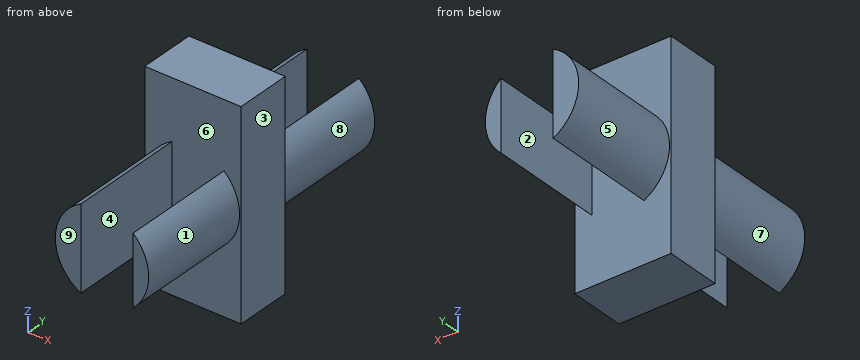
```python
from build123d import *

# Parameters (mm, degrees)
F1_DEPTH = 76.2
F2_W     = 29.7769960016
F2_H     = 106.9766134024
F3_DEPTH = 25.4


with BuildPart() as f1:
    # F0 (on Front) → F1 (new body, symmetric)
    with BuildSketch(Plane.XZ):
        with BuildLine():
            Line((-11.1479088664, -21.9459166651), (-11.1479088664, 21.9459166651))
            ThreePointArc((-11.1479088664, 21.9459166651), (-24.6150183905, 0), (-11.1479088664, -21.9459166651))
        make_face()
    extrude(amount=F1_DEPTH, both=True)



with BuildPart() as f1b:
    # F0 (on Front) → F1, piece 2 (new body, symmetric)
    with BuildSketch(Plane.XZ):
        with BuildLine():
            ThreePointArc((16.3939911872, -18.3612685651), (22.4659467298, -10.0588452567), (24.6150183905, 0))
            ThreePointArc((24.6150183905, 0), (22.4659467298, 10.0588452567), (16.3939911872, 18.3612685651))
            Line((16.3939911872, 18.3612685651), (16.3939911872, -18.3612685651))
        make_face()
    extrude(amount=F1_DEPTH, both=True)


with BuildPart() as f1_1:
    add(f1.part)

    add(f1b.part)  # F3 merges F1b
    # F2 (on Right) → F3 (join, symmetric)
    with BuildSketch(Plane.YZ):
        Rectangle(F2_W, F2_H)
    extrude(amount=F3_DEPTH, both=True)


solid = f1_1.part
```
The listing builds one solid part. Answer for the finished solid, in the listing's coordinates (mm). Face numbers are marked on the shaded views. A direction names the side the tool comes from. Coordinates: 2 decimals unless noted, no trailing zeros. Write each loop counter-clockwise with the first axis right and the second up, starting at its lowest first coordinate (ties: lowest second). Pieces come first, ordered by that corner, then holes. Notation, with made-up numbers: (-35, -6.5) - (-1, -6.5) arc R31 cw to (-1, 27.5) - close; hole circle Ø8 at (82.5, 81.5). An arc over 180 degrees is marked (long way). Return JSON: item names as keys, results as strings. Group by question number.
Q1. Flat-ended cylindrical pins translate along their axes: pin 1 Ø10 at (x, z) = (7, 5) entering from -Y; pin 2 Ø12 at (y, z) = (-48.5, 11) entering from -X; pin 3 Ø11 at (y, z) = (-42.5, -3) entering from -X (3 decimals). Find the tip coordinate at first contact, or state that the pin passes through.
Q2. Which of the six approach directions +Z, -Z, +X, -X, +Y, -Y give full straight-line access (tool end or side, diameter ignored) to the marked faces 1, 2, 3, 4 and 5?
Q3. For a pull along X with two mould halves and no side action, classify the marked faces 6, 7, 8 and 9 as +X half, -X half, draft (parallel to the pull), parting line (faces both ways), or undercut.
Q4. The part is cut by section D-D on z = 5.5. Write down the section's boundary in (x, y).
Q5. The part is cut by section B-B on x = 20. Write down the section's boundary in (y, z), and give its area (3 significant figures).
Q6. The part is cut by section A-A on z = -10.5. Write down the section's boundary in (x, y), and give its area (3 significant figures).
Q7. Find the intervals of material crossed by line 1 along Y through (x, z) = (5, -31.5); line 2 along X through (y, z) = (15, 6); line 3 along X through (y, z) = (-33, -21.5), in increasing order. Write a range as [from, to].
Q8. The part is cut by section C-C on y = 56. Write down the section's boundary in (x, z).
Evaluation:
{
 "1": {"pin 1": "stops at y = -14.89", "pin 2": "stops at x = -24.1", "pin 3": "stops at x = -24.615"},
 "2": {"face 1": "+X, -Y", "face 2": "+Z, -Z, +Y", "face 3": "+Z, -Z, +X, +Y, -Y", "face 4": "+Z, -Z, -Y", "face 5": "-X, +Y"},
 "3": {"face 6": "undercut", "face 7": "-X half", "face 8": "+X half", "face 9": "draft"},
 "4": {"outline": "(-25.4, -14.89) - (-23.99, -14.89) - (-23.99, -76.2) - (-11.15, -76.2) - (-11.15, -14.89) - (16.39, -14.89) - (16.39, -76.2) - (23.99, -76.2) - (23.99, -14.89) - (25.4, -14.89) - (25.4, 14.89) - (23.99, 14.89) - (23.99, 76.2) - (16.39, 76.2) - (16.39, 14.89) - (-11.15, 14.89) - (-11.15, 76.2) - (-23.99, 76.2) - (-23.99, 14.89) - (-25.4, 14.89) - close"},
 "5": {"outline": "(-76.2, -14.35) - (-14.89, -14.35) - (-14.89, -53.49) - (14.89, -53.49) - (14.89, -14.35) - (76.2, -14.35) - (76.2, 14.35) - (14.89, 14.35) - (14.89, 53.49) - (-14.89, 53.49) - (-14.89, 14.35) - (-76.2, 14.35) - close", "area": "6,700 mm2"},
 "6": {"outline": "(-25.4, -14.89) - (-22.26, -14.89) - (-22.26, -76.2) - (-11.15, -76.2) - (-11.15, -14.89) - (16.39, -14.89) - (16.39, -76.2) - (22.26, -76.2) - (22.26, -14.89) - (25.4, -14.89) - (25.4, 14.89) - (22.26, 14.89) - (22.26, 76.2) - (16.39, 76.2) - (16.39, 14.89) - (-11.15, 14.89) - (-11.15, 76.2) - (-22.26, 76.2) - (-22.26, 14.89) - (-25.4, 14.89) - close", "area": "3,600 mm2"},
 "7": {"line 1": "y = [-14.89, 14.89]", "line 2": "x = [-23.87, -11.15], [16.39, 23.87]", "line 3": "x = [-11.99, -11.15]"},
 "8": {"outline": "(-11.15, -21.95) - (-11.15, 21.95) arc R24.62 ccw to start; (16.39, -18.36) arc R24.62 ccw to (16.39, 18.36) - close"}
}
